from build123d import *

# Parameters (mm, degrees)
SKETCH1_W           = 83
SKETCH1_H           = 60
BOSS_EXTRUDE1_DEPTH = 4
SKETCH2_R           = 5
CUT_EXTRUDE1_DEPTH  = 5
SKETCH4_R           = 1.5
CUT_EXTRUDE2_DEPTH  = 10
SKETCH6_R           = 2
CUT_EXTRUDE3_DEPTH  = 10
CUT_EXTRUDE4_DEPTH  = 10
SKETCH8_W           = 4.00000008
SKETCH8_H           = 60
SKETCH8_W_2         = 4
BOSS_EXTRUDE2_DEPTH = 20
FILLET1_R           = 5
SKETCH10_R          = 2
CUT_EXTRUDE5_DEPTH  = 84


with BuildPart() as part:
    # Sketch1 → Boss-Extrude1 (new body)
    with BuildSketch(Plane(origin=(0, 0, 0), x_dir=(0, 0, -1), z_dir=(1, 0, 0))):
        Rectangle(SKETCH1_W, SKETCH1_H)
    extrude(amount=BOSS_EXTRUDE1_DEPTH)

    # Sketch2 → Cut-Extrude1 (cut, through all)
    with BuildSketch(Plane(origin=(4, 0, 0), x_dir=(0, 0, -1), z_dir=(1, 0, 0))):
        Circle(SKETCH2_R)
    extrude(amount=-CUT_EXTRUDE1_DEPTH, mode=Mode.SUBTRACT)

    # Sketch4 → Cut-Extrude2 (cut)
    with BuildSketch(Plane(origin=(4, 0, 0), x_dir=(0, 0, -1), z_dir=(1, 0, 0))):
        with Locations((-13.72367631, 6.054808712)):
            Circle(SKETCH4_R)
        with Locations((-12.105456315, -8.857647962)):
            Circle(SKETCH4_R)
        with Locations((1.618219995, -14.912456674)):
            Circle(SKETCH4_R)
        with Locations((13.72367631, -6.054808712)):
            Circle(SKETCH4_R)
        with Locations((12.105456315, 8.857647962)):
            Circle(SKETCH4_R)
        with Locations((-1.618219995, 14.912456674)):
            Circle(SKETCH4_R)
    extrude(amount=-CUT_EXTRUDE2_DEPTH, mode=Mode.SUBTRACT)

    # Sketch6 → Cut-Extrude3 (cut)
    with BuildSketch(Plane(origin=(4, 0, 0), x_dir=(0, 0, -1), z_dir=(1, 0, 0))):
        with Locations((-26.375, 12.5)):
            Circle(SKETCH6_R)
        with Locations((-26.375, 0)):
            Circle(SKETCH6_R)
        with Locations((-26.375, -12.5)):
            Circle(SKETCH6_R)
        with Locations((26.375, 12.5)):
            Circle(SKETCH6_R)
        with Locations((26.375, 0)):
            Circle(SKETCH6_R)
        with Locations((26.375, -12.5)):
            Circle(SKETCH6_R)
    extrude(amount=-CUT_EXTRUDE3_DEPTH, mode=Mode.SUBTRACT)

    # Sketch7 → Cut-Extrude4 (cut)
    with BuildSketch(Plane(origin=(4, 0, 0), x_dir=(0, 0, -1), z_dir=(1, 0, 0))):
        with BuildLine():
            Line((-19, 23), (-14, 23))
            ThreePointArc((-14, 23), (-12, 21), (-14, 19))
            Line((-14, 19), (-19, 19))
            ThreePointArc((-19, 19), (-21, 21), (-19, 23))
        make_face()
        with BuildLine():
            Line((19, 23), (14, 23))
            ThreePointArc((14, 23), (12, 21), (14, 19))
            Line((14, 19), (19, 19))
            ThreePointArc((19, 19), (21, 21), (19, 23))
        make_face()
    extrude(amount=-CUT_EXTRUDE4_DEPTH, mode=Mode.SUBTRACT)

    # Sketch8 → Boss-Extrude2 (add)
    with BuildSketch(Plane.ZY):
        with Locations((-39.49999996, 0)):
            Rectangle(SKETCH8_W, SKETCH8_H)
        with Locations((39.5, 0)):
            Rectangle(SKETCH8_W_2, SKETCH8_H)
    extrude(amount=BOSS_EXTRUDE2_DEPTH)

    # Fillet1
    fillet1_edges = [part.edges().sort_by_distance(p)[0] for p in [
        (4, 0, -41.5),
        (4, 0, 41.5),
    ]]
    fillet(fillet1_edges, radius=FILLET1_R)

    # Sketch10 → Cut-Extrude5 (cut, through all)
    with BuildSketch(Plane.XY.offset(41.5)):
        with Locations((-12, 15)):
            Circle(SKETCH10_R)
        with Locations((-12, 0)):
            Circle(SKETCH10_R)
        with Locations((-12, -15)):
            Circle(SKETCH10_R)
    extrude(amount=-CUT_EXTRUDE5_DEPTH, mode=Mode.SUBTRACT)


solid = part.part
The model under review builds one solid part; all positions refer to its coordinate system, in mm. A direction names the side the tool comes from. Give positions to 0.01 mm unless a question says otherwise; leave off trailing zeros. Write each loop counter-clockwise with the first axis right and the second up, starting at its lowest first coordinate (ties: lowest second). Pieces come first, ordered by that corner, then holes. Notation, with made-up numbers: M -16.75,49.25 L 36.25,49.25 A15 ccw 36.25,55.25 Z; hole C -40,-2.75 d1. An arc over 180 degrees is marked long. One line per question, with ' | ' between items. Start each with the question number.
Item 1: Wall thickness on line 1 (Z direction, x = -9.25, y = -1.5); line 2 (X direction, y = -19, z = -8); line 3 (Y direction, x = 0.95, z = 0): over which ranges is each line inside the solid? List them lowest first. Write a range as from..to.
Item 2: For faces 1 (the flat face through (2, 23, 17)), 2 (the flat face through (1, 30, 0)), 3 (the flat face through (0, -6, 1)), list the 3-axis set-ups (+Z, -Z, +X, -X, +Y, -Y) from which the entire face can be reached by the end or side of a thin tool; tool diameter is ignored.
Item 3: Draft analysis for pull direction Z (two halves, no side actions). For faces 4 (the cylindrical face through (2, 21, 12)), 5 (the cylindrical face through (2, 21, 21)), 6 (the cylindrical face through (2.5, 0.42, -40.07)), 7 (the flat face through (-20, 0, -40)), state which applies: released by +Z, released by -Z, zero draft, split by the parting line, or undercut.
Item 4: For pin 1 (4 mm diameter, centred on y = -8.86, z = 12.11, fed in from -X), flat-tipped, find the tip position at first contact; note if it passes through.
Item 5: We need section B-B on z = 17.5. Write out the cut boundary in (x, y), plus the area to 3 significant figures.
Item 6: We need section C-C on x = -12. Give the number of separate pieces and of enclosed holes in the cut face, plus the area to 3 significant figures.
Item 7: We need section D-D on y = -25.5. Write out the cut boundary in (x, z), plus the area to 3 significant figures.
Item 8: We need section A-A on x = -17. Write out the cut boundary in (y, z).
Results found:
1) line 1: z = -41.5..-37.5, 37.5..41.5 | line 2: x = 0..4 | line 3: y = -30..-5, 5..30
2) face 1: +X, -X | face 2: +Z, -Z, +X, -X, +Y | face 3: -X, +Y, -Y
3) face 4: undercut | face 5: undercut | face 6: released by -Z | face 7: zero draft
4) pin 1: stops at x = 0
5) outline: M 0,-30 L 4,-30 L 4,19 L 0,19 Z; M 0,23 L 4,23 L 4,30 L 0,30 Z | area: 224 mm2
6) separate pieces: 8 | enclosed holes: 0 | area: 384 mm2
7) outline: M -20,-41.5 L -1,-41.5 A5 ccw 4,-36.5 L 4,36.5 A5 ccw -1,41.5 L -20,41.5 L -20,37.5 L 0,37.5 L 0,-37.5 L -20,-37.5 Z | area: 481 mm2
8) outline: M -30,-41.5 L 30,-41.5 L 30,-37.5 L -30,-37.5 Z; M -30,37.5 L 30,37.5 L 30,41.5 L -30,41.5 Z
